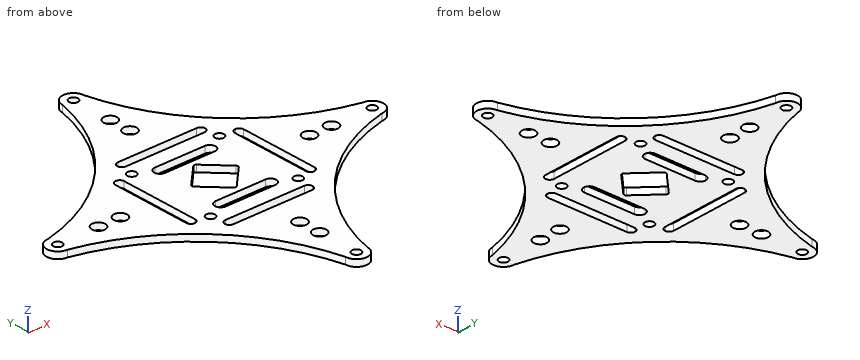
from build123d import *

# Parameters (mm, degrees)
MODEL_R         = 1
MODEL_R_2       = 1.5
EXTRUDE_1_DEPTH = 1.5


with BuildPart() as part:
    # Model → 凸台-拉伸1 (new body)
    with BuildSketch(Plane.XY):
        with BuildLine():
            ThreePointArc((52.402811695, 15.581837899), (64.310189073, 37.053271897), (85.771502284, 48.978880864))
            ThreePointArc((85.771502284, 48.978880864), (88.271502284, 51.478880864), (85.771502284, 53.978880864))
            ThreePointArc((85.771502284, 53.978880864), (64.310189073, 65.90448983), (52.402811695, 87.375923829))
            ThreePointArc((52.402811695, 87.375923829), (49.902811695, 89.875923829), (47.402811695, 87.375923829))
            ThreePointArc((47.402811695, 87.375923829), (35.495434317, 65.90448983), (14.034121106, 53.978880864))
            ThreePointArc((14.034121106, 53.978880864), (11.534121106, 51.478880864), (14.034121106, 48.978880864))
            ThreePointArc((14.034121106, 48.978880864), (35.495434317, 37.053271897), (47.402811695, 15.581837899))
            ThreePointArc((47.402811695, 15.581837899), (49.902811695, 13.081837899), (52.402811695, 15.581837899))
        make_face()
        with Locations((39.902811695, 41.478880864)):
            Circle(MODEL_R, mode=Mode.SUBTRACT)
        with BuildLine():
            Line((37.266458229, 60.471548336), (37.266458229, 42.471548336))
            ThreePointArc((37.266458229, 42.471548336), (36.97356501, 41.764441555), (36.266458229, 41.471548336))
            ThreePointArc((36.266458229, 41.471548336), (35.559351447, 41.764441555), (35.266458229, 42.471548336))
            Line((35.266458229, 42.471548336), (35.266458229, 60.471548336))
            ThreePointArc((35.266458229, 60.471548336), (36.266458229, 61.471548336), (37.266458229, 60.471548336))
        make_face(mode=Mode.SUBTRACT)
        with BuildLine():
            ThreePointArc((55.514109326, 44.893015049), (56.787629095, 43.61949528), (55.514109326, 42.34597551))
            Line((55.514109326, 42.34597551), (44.120323024, 42.345975511))
            ThreePointArc((44.120323024, 42.345975511), (43.219808559, 42.718980816), (42.846803254, 43.619495281))
            ThreePointArc((42.846803254, 43.619495281), (43.219808559, 44.520009746), (44.120323024, 44.89301505))
            Line((44.120323024, 44.89301505), (55.514109326, 44.893015049))
        make_face(mode=Mode.SUBTRACT)
        with Locations((49.902811695, 15.581837899)):
            Circle(MODEL_R, mode=Mode.SUBTRACT)
        with Locations((49.902811695, 24.912124037)):
            Circle(MODEL_R_2, mode=Mode.SUBTRACT)
        with Locations((49.902811695, 29.912124037)):
            Circle(MODEL_R_2, mode=Mode.SUBTRACT)
        with BuildLine():
            Line((58.895479167, 38.842527397), (58.910144223, 38.842527397))
            ThreePointArc((58.910144223, 38.842527397), (59.617251004, 38.549634178), (59.910144223, 37.842527397))
            ThreePointArc((59.910144223, 37.842527397), (59.617251004, 37.135420616), (58.910144223, 36.842527397))
            Line((58.910144223, 36.842527397), (58.895479167, 36.842527397))
            Line((58.895479167, 36.842527397), (40.910144223, 36.842527397))
            Line((40.910144223, 36.842527397), (40.895479167, 36.842527397))
            ThreePointArc((40.895479167, 36.842527397), (40.188372386, 37.135420616), (39.895479167, 37.842527397))
            ThreePointArc((39.895479167, 37.842527397), (40.188372386, 38.549634178), (40.895479167, 38.842527397))
            Line((40.895479167, 38.842527397), (40.910144223, 38.842527397))
            Line((40.910144223, 38.842527397), (58.895479167, 38.842527397))
        make_face(mode=Mode.SUBTRACT)
        with Locations((59.902811695, 41.478880864)):
            Circle(MODEL_R, mode=Mode.SUBTRACT)
        with Locations((14.034121106, 51.478880864)):
            Circle(MODEL_R, mode=Mode.SUBTRACT)
        with Locations((23.336054869, 51.478880864)):
            Circle(MODEL_R_2, mode=Mode.SUBTRACT)
        with Locations((28.336054869, 51.478880864)):
            Circle(MODEL_R_2, mode=Mode.SUBTRACT)
        with Locations((39.902811695, 61.478880864)):
            Circle(MODEL_R, mode=Mode.SUBTRACT)
        with BuildLine():
            Line((58.895479167, 64.11523433), (40.895479167, 64.11523433))
            ThreePointArc((40.895479167, 64.11523433), (40.188372386, 64.408127549), (39.895479167, 65.11523433))
            ThreePointArc((39.895479167, 65.11523433), (40.188372386, 65.822341111), (40.895479167, 66.11523433))
            Line((40.895479167, 66.11523433), (58.895479167, 66.11523433))
            ThreePointArc((58.895479167, 66.11523433), (59.895479167, 65.11523433), (58.895479167, 64.11523433))
        make_face(mode=Mode.SUBTRACT)
        with BuildLine():
            Line((50.256365086, 56.590224257), (55.014155089, 51.832434254))
            ThreePointArc((55.014155089, 51.832434254), (55.160601698, 51.478880864), (55.014155089, 51.125327473))
            Line((55.014155089, 51.125327473), (50.256365086, 46.36753747))
            ThreePointArc((50.256365086, 46.36753747), (49.902811695, 46.221090861), (49.549258305, 46.36753747))
            Line((49.549258305, 46.36753747), (44.791468302, 51.125327473))
            ThreePointArc((44.791468302, 51.125327473), (44.645021692, 51.478880864), (44.791468302, 51.832434254))
            Line((44.791468302, 51.832434254), (49.549258305, 56.590224257))
            ThreePointArc((49.549258305, 56.590224257), (49.902811695, 56.736670867), (50.256365086, 56.590224257))
        make_face(mode=Mode.SUBTRACT)
        with BuildLine():
            Line((44.321526015, 60.538332308), (55.715312317, 60.538332308))
            ThreePointArc((55.715312317, 60.538332308), (56.988832087, 59.264812538), (55.715312317, 57.991292769))
            Line((55.715312317, 57.991292769), (44.321526015, 57.991292769))
            ThreePointArc((44.321526015, 57.991292769), (43.42101155, 58.364298073), (43.048006246, 59.264812538))
            ThreePointArc((43.048006246, 59.264812538), (43.42101155, 60.165327003), (44.321526015, 60.538332308))
        make_face(mode=Mode.SUBTRACT)
        with BuildLine():
            Line((62.539165162, 42.486213392), (62.539165162, 60.486213392))
            ThreePointArc((62.539165162, 60.486213392), (62.832058381, 61.193320173), (63.539165162, 61.486213392))
            ThreePointArc((63.539165162, 61.486213392), (64.246271943, 61.193320173), (64.539165162, 60.486213392))
            Line((64.539165162, 60.486213392), (64.539165162, 42.486213392))
            ThreePointArc((64.539165162, 42.486213392), (63.539165162, 41.486213392), (62.539165162, 42.486213392))
        make_face(mode=Mode.SUBTRACT)
        with Locations((59.902811695, 61.478880864)):
            Circle(MODEL_R, mode=Mode.SUBTRACT)
        with Locations((71.469568521, 51.478880864)):
            Circle(MODEL_R_2, mode=Mode.SUBTRACT)
        with Locations((76.469568521, 51.478880864)):
            Circle(MODEL_R_2, mode=Mode.SUBTRACT)
        with Locations((85.771502284, 51.478880864)):
            Circle(MODEL_R, mode=Mode.SUBTRACT)
        with Locations((49.902811695, 73.04563769)):
            Circle(MODEL_R_2, mode=Mode.SUBTRACT)
        with Locations((49.902811695, 78.04563769)):
            Circle(MODEL_R_2, mode=Mode.SUBTRACT)
        with Locations((49.902811695, 87.375923829)):
            Circle(MODEL_R, mode=Mode.SUBTRACT)
    extrude(amount=EXTRUDE_1_DEPTH)


solid = part.part
CAD build for the part. Positions are in the model's coordinates, mm. Round coordinates to 2 decimals unless told otherwise and drop trailing zeros. Loops run counter-clockwise (first coordinate to the right, second up) from the corner with the lowest first, then second, coordinate; pieces in that order, holes last.
(1) Cut at D-D (x = 79.5). Give the cut face in (y, z), plus the area to 3 significant figures.
(2) Drop flat-ended pins along their axis: pin 1 (1.8 mm diameter, centred on x = 76.47, y = 51.48, fed in from -Z); pin 2 (0.8 mm diameter, centred on x = 48.5, z = 1, fed in from +Y); pin 3 (0.8 mm diameter, centred on x = 47.5, z = 1, fed in from -Y); pin 4 (0.8 mm diameter, centred on y = 52.5, z = 0.5, fed in from +X). Give the stop position or say it passes through.
(3) Cut at C-C (z = 0.55). State how many separate pieces and enclosed holes the cut face has, plus the area to 3 significant figures.
(4) Cut at A-A (x = 46). Give the cut face in (y, z).
(5) Wall check: line 1 along Y through (x, z) = (45, 1); line 2 along X through (y, z) = (45.5, 0.3); line 3 along Y through (x, z) = (59.5, 0.6). Give the ranges that are in metal, low to high.
(6) Cut at B-B (y = 33.5). Give the cut face in (x, z), plus the area to 3 significant figures.
Findings below:
1. outline: (47.02, 0) - (55.93, 0) - (55.93, 1.5) - (47.02, 1.5) - close
1. area: 13.4 mm2
2. pin 1: passes through
2. pin 2: stops at y = 89.67
2. pin 3: stops at y = 14.09
2. pin 4: stops at x = 88.19
3. separate pieces: 1
3. enclosed holes: 23
3. area: 1,730 mm2
4. outline: (20.39, 0) - (36.84, 0) - (36.84, 1.5) - (20.39, 1.5) - close; (38.84, 0) - (42.35, 0) - (42.35, 1.5) - (38.84, 1.5) - close; (44.89, 0) - (49.92, 0) - (49.92, 1.5) - (44.89, 1.5) - close; (53.04, 0) - (57.99, 0) - (57.99, 1.5) - (53.04, 1.5) - close; (60.54, 0) - (64.12, 0) - (64.12, 1.5) - (60.54, 1.5) - close; (66.12, 0) - (82.57, 0) - (82.57, 1.5) - (66.12, 1.5) - close
5. line 1: y = 22.96 to 36.84, 38.84 to 42.35, 44.89 to 50.92, 52.04 to 57.99, 60.54 to 64.12, 66.12 to 80
5. line 2: x = 23.74 to 35.27, 37.27 to 62.54, 64.54 to 76.07
5. line 3: y = 31.36 to 37.04, 38.65 to 40.56, 42.39 to 60.56, 62.39 to 64.32, 65.91 to 71.6
6. outline: (38.68, 0) - (61.12, 0) - (61.12, 1.5) - (38.68, 1.5) - close
6. area: 33.7 mm2
